Could you check a few things on this drawing? It's one solid part, dimensions in mm from its lowest x, y, z. A direction names the side the tool comes from. Round coordinates to 2 decimals unless told otherwise and drop trailing zeros. Write each loop counter-clockwise with the first axis right and the second up, starting at its lowest first coordinate (ties: lowest second). Pieces come first, ordered by that corner, then holes. Notation, with made-up numbers: M 43.25,8 L 90.25,8 A22 ccw 90.25,22 Z; hole C -39,-34 d4. An arc over 180 degrees is marked long. One line per item, written item: value. Start each with the question number.
(1) If I drill on L1, parallel to Y at x = 6, z = 28; L2, parallel to X at y = 84, z = 25.5; L3, parallel to Z at x = 11, y = 38, over which ranges is the centre line in solid material (lowest first)?
(2) I want a section at B-B on x = 16. Please give me the cut outline in (y, z).
(3) I want a section at C-C on y = 31. Please give me the cut outline in (x, z), and give its area (3 significant figures).
(4) Which directions (+Z, -Z, +X, -X, +Y, -Y) give clear straight access to the entire face, cutting with the end or side of a thin tool? Please do the marked faces 1, 2 and 3.
(5) I want a section at A-A on z = 16. Please give me the cut outline in (x, y), and give its area (3 significant figures).
(6) I'm going to push flat-ended pins straight in: pin 1 Ø8 at (x, y) = (9, 72) entering from -Z; pin 2 Ø5 at (x, y) = (24.5, 39) entering from -Z; pin 3 Ø3 at (y, z) = (18.5, 8.5) entering from -X. Where does each tip first touch, or does it pass through?
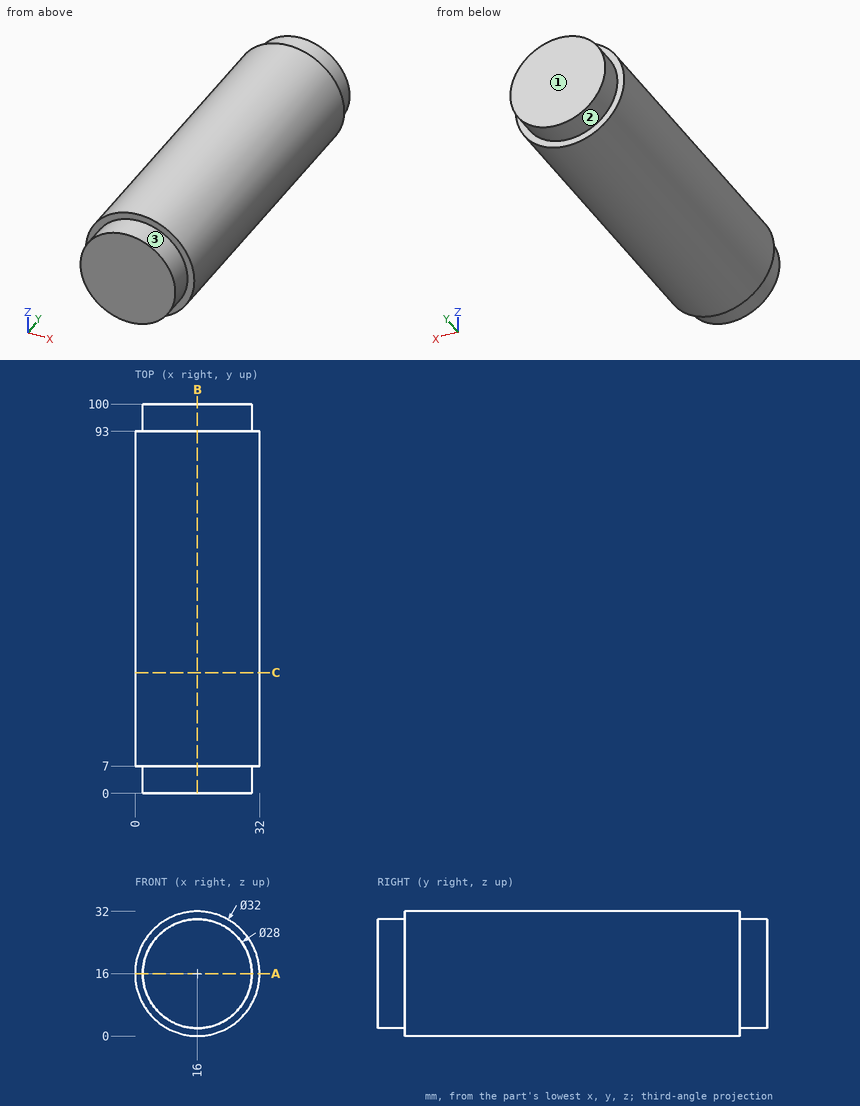
Found:
1. L1: y = 7 to 93
1. L2: x = 3.13 to 28.87
1. L3: z = 0.8 to 31.2
2. outline: M 0,2 L 7,2 L 7,0 L 93,0 L 93,2 L 100,2 L 100,30 L 93,30 L 93,32 L 7,32 L 7,30 L 0,30 Z
3. outline: C 16,16 d32
3. area: 804 mm²
4. face 1: +Z, -Z, +X, -X, +Y
4. face 2: +Y
4. face 3: -Y
5. outline: M 0,7 L 2,7 L 2,0 L 30,0 L 30,7 L 32,7 L 32,93 L 30,93 L 30,100 L 2,100 L 2,93 L 0,93 Z
5. area: 3,140 mm²
6. pin 1: stops at z = 0.28
6. pin 2: stops at z = 1.17
6. pin 3: stops at x = 1.17
